The listing builds one solid part. Answer for the finished solid, in the listing's coordinates (mm). Face numbers are marked on the shaded views. A direction names the side the tool comes from. Give positions to 0.01 mm unless a question says otherwise; leave off trailing zeros. Write each loop counter-clockwise with the first axis right and the second up, starting at its lowest first coordinate (ties: lowest second). Pieces come first, ordered by that corner, then holes. Notation, with made-up numbers: (-3, 6.25) - (34, 6.25) arc R35 cw to (34, 44.25) - close; hole circle Ø11 at (19, -7). An arc over 180 degrees is marked (long way). One line per item, written item: value. Start each with the question number.
from build123d import *

# Parameters (mm, degrees)
SKETCH1_7_W         = 63
SKETCH1_7_H         = 55
SKETCH1_7_R         = 1.5
SKETCH1_7_R_2       = 8.375
BOSS_EXTRUDE3_DEPTH = 7
BOSS_EXTRUDE4_START = -45
SKETCH1_8_W         = 63
SKETCH1_8_H         = 55
SKETCH1_8_R         = 1.5
SKETCH1_8_W_2       = 43
SKETCH1_8_H_2       = 43
BOSS_EXTRUDE4_DEPTH = 45
SKETCH1_9_R         = 8.375
SKETCH1_9_R_2       = 6.75
BOSS_EXTRUDE5_DEPTH = 5
SKETCH4_W           = 12.5
SKETCH4_H           = 45
CUT_EXTRUDE5_DEPTH  = 6


with BuildPart() as part:
    # Sketch1<7> → Boss-Extrude3 (new body)
    with BuildSketch(Plane.XY):
        with Locations((21.5, 21.5)):
            Rectangle(SKETCH1_7_W, SKETCH1_7_H)
        with Locations((-5, 36.5)):
            Circle(SKETCH1_7_R, mode=Mode.SUBTRACT)
        with Locations((-5, 6.5)):
            Circle(SKETCH1_7_R, mode=Mode.SUBTRACT)
        with Locations((48, 6.5)):
            Circle(SKETCH1_7_R, mode=Mode.SUBTRACT)
        with Locations((48, 36.5)):
            Circle(SKETCH1_7_R, mode=Mode.SUBTRACT)
        with Locations((21.5, 21.5)):
            Circle(SKETCH1_7_R_2, mode=Mode.SUBTRACT)
    extrude(amount=BOSS_EXTRUDE3_DEPTH)

    # Sketch1<8> → Boss-Extrude4 (add)
    with BuildSketch(Plane.XY.offset(BOSS_EXTRUDE4_START)):
        with Locations((21.5, 21.5)):
            Rectangle(SKETCH1_8_W, SKETCH1_8_H)
        with Locations((48, 6.5)):
            Circle(SKETCH1_8_R, mode=Mode.SUBTRACT)
        with Locations((-5, 6.5)):
            Circle(SKETCH1_8_R, mode=Mode.SUBTRACT)
        with Locations((-5, 36.5)):
            Circle(SKETCH1_8_R, mode=Mode.SUBTRACT)
        with Locations((48, 36.5)):
            Circle(SKETCH1_8_R, mode=Mode.SUBTRACT)
        with Locations((21.5, 21.5)):
            Rectangle(SKETCH1_8_W_2, SKETCH1_8_H_2, mode=Mode.SUBTRACT)
    extrude(amount=BOSS_EXTRUDE4_DEPTH)

    # Sketch1<9> → Boss-Extrude5 (add)
    with BuildSketch(Plane.XY):
        with Locations((21.5, 21.5)):
            Circle(SKETCH1_9_R)
        with Locations((21.5, 21.5)):
            Circle(SKETCH1_9_R_2, mode=Mode.SUBTRACT)
    extrude(amount=BOSS_EXTRUDE5_DEPTH)

    # Sketch4 → Cut-Extrude5 (cut)
    with BuildSketch(Plane.XZ.offset(-43)):
        with Locations((27.75, -22.5)):
            Rectangle(SKETCH4_W, SKETCH4_H)
        with Locations((15.25, -22.5)):
            Rectangle(SKETCH4_W, SKETCH4_H)
    extrude(amount=-CUT_EXTRUDE5_DEPTH, mode=Mode.SUBTRACT)


solid = part.part
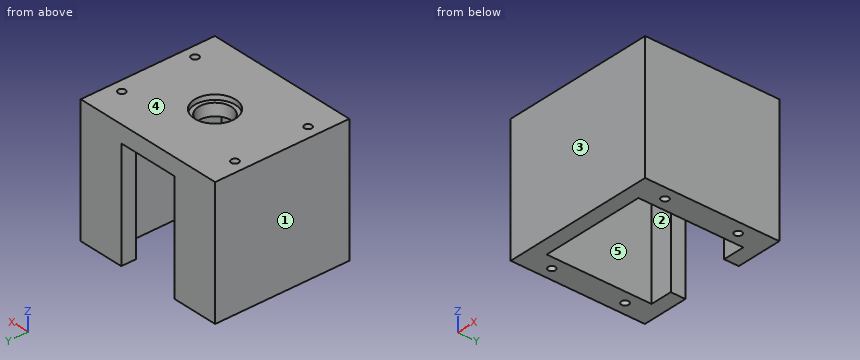
Item 1: Find section A-A on x = 21.5. Determine the outline of the cut face in (y, z) (3 decimals).
Item 2: Find section C-C on z = -25.5. Determine the outline of the cut face in (x, y), plus the area to 3 significant figures.
Item 3: Find section B-B on y = 21.5. Determine the outline of the cut face in (x, z) (3 decimals).
Item 4: For the marked faces 4 and 5, determine the directions among +Z, -Z, +X, -X, +Y, -Y from which every point of the face is accessible in a straight line to the end or side of a thin tool.
Item 5: Find section D-D on x = 48. Determine the outline of the cut face in (y, z), plus the area to 3 significant figures.
Item 6: Straight lines are drawn through the part: line 1 along Y through (x, z) = (-5, -30.5); line 2 along Y through (x, z) = (21, 3); line 3 along X through (y, z) = (39, -20.5). For each, find the intervals that lie inside material, in ascending order.
Item 7: This flat-tipped pin is pushed along its axis until it touches: pin 1 Ø15.5 at (x, y) = (21.5, 21.5) entering from +Z. Where does it stop, or does it pass through?
Item 8: The mould has two halves that part along X. Classify the marked faces 1, 2 and 3: +X half, -X half, draft (parallel to the pull), parting line (faces both ways), or undercut.
Values:
1. outline: (-6, -45) - (0, -45) - (0, 0) - (14.75, 0) - (14.75, 5) - (13.125, 5) - (13.125, 7) - (-6, 7) - close; (28.25, 0) - (49, 0) - (49, 7) - (29.875, 7) - (29.875, 5) - (28.25, 5) - close
2. outline: (-10, -6) - (53, -6) - (53, 49) - (34, 49) - (34, 43) - (43, 43) - (43, 0) - (0, 0) - (0, 43) - (9, 43) - (9, 49) - (-10, 49) - close; hole circle Ø3 at (-5, 6.5); hole circle Ø3 at (-5, 36.5); hole circle Ø3 at (48, 6.5); hole circle Ø3 at (48, 36.5)
2. area: 1,440 mm^2
3. outline: (-10, -45) - (0, -45) - (0, 0) - (14.75, 0) - (14.75, 5) - (13.125, 5) - (13.125, 7) - (-10, 7) - close; (28.25, 0) - (43, 0) - (43, -45) - (53, -45) - (53, 7) - (29.875, 7) - (29.875, 5) - (28.25, 5) - close
4. face 4: +Z, +X, -X, +Y, -Y
4. face 5: -Z
5. outline: (-6, -45) - (5, -45) - (5, 7) - (-6, 7) - close; (8, -45) - (35, -45) - (35, 7) - (8, 7) - close; (38, -45) - (49, -45) - (49, 7) - (38, 7) - close
5. area: 2,550 mm^2
6. line 1: -6 to 5, 8 to 35, 38 to 49
6. line 2: -6 to 14.77, 28.23 to 49
6. line 3: -10 to 0, 43 to 53
7. pin 1: z = 5
8. face 1: -X half
8. face 2: undercut
8. face 3: draft
